Design review of the part built by this model. Coordinates are the model's own, in mm. A direction names the side the tool comes from. Coordinates: 2 decimals unless noted, no trailing zeros. Loops run counter-clockwise (first coordinate to the right, second up) from the corner with the lowest first, then second, coordinate; pieces in that order, holes last. Notation, with made-up numbers: M -20.5,31 L -14.5,31 A22 ccw -14.5,50 Z; hole C 89,25.5 d4. An arc over 180 degrees is marked long. Write item = value, one per line. Start each with the question number.
```python
from build123d import *

# Parameters (mm, degrees)
SKETCH1_R           = 1.75
SKETCH1_R_2         = 1.798521792
BOSS_EXTRUDE1_DEPTH = 10
SKETCH2_R           = 2.65
CUT_EXTRUDE1_DEPTH  = 3.5


with BuildPart() as part:
    # Sketch1 → Boss-Extrude1 (new body)
    with BuildSketch(Plane.YZ):
        Polygon((-45, -15.65), (-45, 15.65), (-38.3, 22.35), (-29.12737367, 22.35), (-21.9, 29.57737367), (-21.9, 35.8), (-15.2, 42.5), (15.2, 42.5), (21.9, 35.8), (21.9, 29.57737367), (29.12737367, 22.35), (38.3, 22.35), (45, 15.65), (45, -15.65), (38.3, -22.35), (29.12737367, -22.35), (21.9, -29.57737367), (21.9, -35.8), (15.2, -42.5), (-15.2, -42.5), (-21.9, -35.8), (-21.9, -29.57737367), (-29.12737367, -22.35), (-38.3, -22.35), align=None)
        with Locations(Location((0, 32.15, 0), (0, 0, 270))):
            Circle(SKETCH1_R, mode=Mode.SUBTRACT)
        with Locations(Location((-32.15, 0, 0), (0, 0, 270))):
            Circle(SKETCH1_R, mode=Mode.SUBTRACT)
        with Locations(Location((0, -32.15, 0), (0, 0, 270))):
            Circle(SKETCH1_R, mode=Mode.SUBTRACT)
        with Locations(Location((32.15, 0, 0), (0, 0, 270))):
            Circle(SKETCH1_R, mode=Mode.SUBTRACT)
        with Locations(Location((-15, 30, 0), (0, 0, 270))):
            Circle(SKETCH1_R_2, mode=Mode.SUBTRACT)
        with Locations(Location((15, 30, 0), (0, 0, 270))):
            Circle(SKETCH1_R_2, mode=Mode.SUBTRACT)
        with Locations(Location((15, -30, 0), (0, 0, 270))):
            Circle(SKETCH1_R_2, mode=Mode.SUBTRACT)
        with Locations(Location((-15, -30, 0), (0, 0, 270))):
            Circle(SKETCH1_R_2, mode=Mode.SUBTRACT)
    extrude(amount=BOSS_EXTRUDE1_DEPTH)

    # Sketch2 → Cut-Extrude1 (cut)
    with BuildSketch(Plane(origin=(0, 0, 0), x_dir=(0, -1, 0), z_dir=(-1, 0, 0))):
        with Locations(Location((-15, 30, 0), (0, 0, 90))):
            Circle(SKETCH2_R)
        with Locations(Location((15, 30, 0), (0, 0, 90))):
            Circle(SKETCH2_R)
        with Locations(Location((15, -30, 0), (0, 0, 90))):
            Circle(SKETCH2_R)
        with Locations(Location((-15, -30, 0), (0, 0, 90))):
            Circle(SKETCH2_R)
    extrude(amount=-CUT_EXTRUDE1_DEPTH, mode=Mode.SUBTRACT)


solid = part.part
```
(1) To check wall thickness, follow L1, parallel to Y at x = 5.25, z = -30; L2, parallel to Y at x = 1.65, z = -30; L3, parallel to Z at x = 2, y = -17. State the ranges of each line that lie inside material, in increasing order.
(2) Take a section at B-B (x = 6.5). Give the number of separate pieces and of enclosed holes in the cut face, plus the area to 3 significant figures.
(3) Take a section at C-C (z = -25.5). State the section outline as (x, y) points.
(4) Insertion check: pin 1 (4 mm diameter, centred on y = -15, z = 30, fed in from -X); pin 2 (3 mm diameter, centred on x = 5, z = 32, fed in from -Y); pin 3 (3 mm diameter, centred on x = 8, z = -34, fed in from +Y). Each pin has a flat end and moves straight along its axis. Give the tip position at first contact, or say it passes through.
(5) Mouldability with a two-part tool opening along Z and no side actions: class faces 4 (the flat face through (3.5, 13, -29)), 5 (the flat face through (5, 0, -42.5)), 6 (the flat face through (4.9, -18.6, 39.1)), 7 (the cylindrical face through (1.726, 15.117, -32.647)) as +Z half, -Z half, draft (parallel to the pull), parting line (faces both ways), or undercut.
(6) Tool access review of faces 1 (the flat face through (5, -21.9, -33)), 2 (the flat face through (5, 21.9, -33)), 3 (the flat face through (5, -34, 22.35)): name each direction out of +Z, -Z, +X, -X, +Y, -Y from which nothing blocks a thin tool from reaching the whole face with its end or side.
(7) Take a section at A-A (y = -32.15). State the section outline as (x, z) points.
Results list:
q1.L1 = -21.9 to -16.8, -13.2 to 13.2, 16.8 to 21.9
q1.L2 = -21.9 to -17.65, -12.35 to 12.35, 17.65 to 21.9
q1.L3 = -40.7 to -31.74, -28.26 to 28.26, 31.74 to 40.7
q2.separate_pieces = 1
q2.enclosed_holes = 8
q2.area = 5,630 mm^2
q3.outline = M 0,-25.98 L 10,-25.98 L 10,25.98 L 0,25.98 Z
q4.pin_1 = 3.5
q4.pin_2 = -21.9
q4.pin_3 = 21.9
q5.face_4 = undercut
q5.face_5 = -Z half
q5.face_6 = +Z half
q5.face_7 = undercut
q6.face_1 = -Z, +X, -X, -Y
q6.face_2 = -Z, +X, -X, +Y
q6.face_3 = +Z, +X, -X, -Y
q7.outline = M 0,-22.35 L 10,-22.35 L 10,-1.75 L 0,-1.75 Z; M 0,1.75 L 10,1.75 L 10,22.35 L 0,22.35 Z
